Can you work these out from the model? Positions are in its coordinate system, mm. Face numbers are marked on the shaded views. A direction names the side the tool comes from. Coordinates: 2 decimals unless noted, no trailing zeros. Write each loop counter-clockwise with the first axis right and the second up, starting at its lowest first coordinate (ties: lowest second). Pieces come first, ordered by that corner, then holes.
```python
from build123d import *

# Parameters (mm, degrees)
SKETCH1_R           = 5.05
BOSS_EXTRUDE1_DEPTH = 6.35
SKETCH2_W           = 10
SKETCH2_H           = 20
BOSS_EXTRUDE2_DEPTH = 50


with BuildPart() as part:
    # Sketch1 → Boss-Extrude1 (new body)
    with BuildSketch(Plane(origin=(0, 0, 0), x_dir=(1, 0, 0), z_dir=(0, 1, 0))):
        Polygon((45, 75), (-50, 75), (-50, 67.7), (-50, 47.7), (-50, -47.7), (-50, -67.7), (-50, -75), (45, -75), align=None)
        with Locations(Location((-36, 26, 0), (0, 0, 270))):
            Circle(SKETCH1_R, mode=Mode.SUBTRACT)
        with Locations(Location((36, 26, 0), (0, 0, 270))):
            Circle(SKETCH1_R, mode=Mode.SUBTRACT)
        with Locations(Location((36, -26, 0), (0, 0, 270))):
            Circle(SKETCH1_R, mode=Mode.SUBTRACT)
        with Locations(Location((-36, -26, 0), (0, 0, 270))):
            Circle(SKETCH1_R, mode=Mode.SUBTRACT)
        with Locations(Location((0, 26, 0), (0, 0, 270))):
            Circle(SKETCH1_R, mode=Mode.SUBTRACT)
        with Locations(Location((0, -26, 0), (0, 0, 270))):
            Circle(SKETCH1_R, mode=Mode.SUBTRACT)
    extrude(amount=BOSS_EXTRUDE1_DEPTH)

    # Sketch2 → Boss-Extrude2 (add)
    with BuildSketch(Plane(origin=(0, 0, 0), x_dir=(1, 0, 0), z_dir=(0, 1, 0))):
        with Locations((-55, 44.5)):
            Rectangle(SKETCH2_W, SKETCH2_H)
        with Locations((-55, -44.5)):
            Rectangle(SKETCH2_W, SKETCH2_H)
    extrude(amount=BOSS_EXTRUDE2_DEPTH)


solid = part.part
```
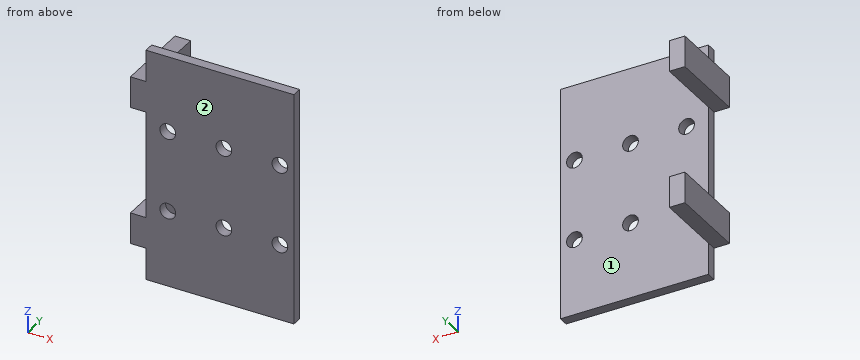
1. I'm going to push flat-ended pins straight in: P1, Ø3, axis at x = -53, y = 18.5, coming from the +Z side; P2, Ø16, axis at y = 28, z = -49.5, coming from the +X side; P3, Ø6, axis at x = 0, z = -26, coming from the -Y side; P4, Ø13, axis at x = -36, z = -26, coming from the +Y side. Where does each tip first touch, or does it pass through?
2. If we section it at D-D, the plane z = -50.5: List the corners of the cut face in (x, y) for me.
3. If we section it at A-A, the plane x = 36: List the corners of the cut face in (y, z) for me.
4. If we section it at C-C, the plane y = 16: List the corners of the cut face in (x, z) for me.
5. If we section it at B-B, the plane z = 26: List the corners of the cut face in (x, y) for me, plus the area to 3 significant figures.
6. Which directions (+Z, -Z, +X, -X, +Y, -Y) give clear straight access to the entire face, cutting with the end or side of a thin tool? Please do the marked faces 1 and 2.
7. If I drill on L1, parallel to X at y = 5.25, z = 26; L2, parallel to Z at x = -52, y = 6; L3, parallel to Y at x = -42, z = 43, over which ranges is the centre line in solid material (lowest first)?
Answers:
1. P1: stops at z = 54.5
1. P2: stops at x = -50
1. P3: passes through
1. P4: stops at y = 6.35
2. outline: (-60, 0) - (45, 0) - (45, 6.35) - (-50, 6.35) - (-50, 50) - (-60, 50) - close
3. outline: (0, -75) - (6.35, -75) - (6.35, -31.05) - (0, -31.05) - close; (0, -20.95) - (6.35, -20.95) - (6.35, 20.95) - (0, 20.95) - close; (0, 31.05) - (6.35, 31.05) - (6.35, 75) - (0, 75) - close
4. outline: (-60, -54.5) - (-50, -54.5) - (-50, -34.5) - (-60, -34.5) - close; (-60, 34.5) - (-50, 34.5) - (-50, 54.5) - (-60, 54.5) - close
5. outline: (-50, 0) - (-41.05, 0) - (-41.05, 6.35) - (-50, 6.35) - close; (-30.95, 0) - (-5.05, 0) - (-5.05, 6.35) - (-30.95, 6.35) - close; (5.05, 0) - (30.95, 0) - (30.95, 6.35) - (5.05, 6.35) - close; (41.05, 0) - (45, 0) - (45, 6.35) - (41.05, 6.35) - close
5. area: 411 mm2
6. face 1: +Z, -Z, +X, +Y
6. face 2: +Z, -Z, +X, -X, -Y
7. L1: x = -50 to -41.05, -30.95 to -5.05, 5.05 to 30.95, 41.05 to 45
7. L2: z = -54.5 to -34.5, 34.5 to 54.5
7. L3: y = 0 to 6.35
